from build123d import *

# Parameters (mm, degrees)
F0_R     = 1.5
F0_R_2   = 2.5
F1_DEPTH = 5
F2_R     = 2.5


with BuildPart() as f1:
    # F0 (on Front) → F1 (new body)
    with BuildSketch(Plane.XZ):
        with BuildLine():
            Line((-20, -25), (20, -25))
            ThreePointArc((20, -25), (27.071068, -22.071068), (30, -15))
            Line((30, -15), (30, 15))
            ThreePointArc((30, 15), (27.071068, 22.071068), (20, 25))
            Line((20, 25), (-20, 25))
            ThreePointArc((-20, 25), (-27.071068, 22.071068), (-30, 15))
            Line((-30, 15), (-30, -15))
            ThreePointArc((-30, -15), (-27.071068, -22.071068), (-20, -25))
        make_face()
        with Locations((-6, -20.123001)):
            Circle(F0_R, mode=Mode.SUBTRACT)
        with Locations((6, -20.123001)):
            Circle(F0_R, mode=Mode.SUBTRACT)
        with Locations((-10, 0)):
            Circle(F0_R_2, mode=Mode.SUBTRACT)
        with Locations((10, 0)):
            Circle(F0_R_2, mode=Mode.SUBTRACT)
    extrude(amount=F1_DEPTH)

    # F2
    f2_edges = [f1.edges().sort_by_distance(p)[0] for p in [
        (-30, -5, 0),
        (30, -5, 0),
        (0, -5, 25),
        (0, -5, -25),
        (-27.071068, -5, -22.071068),
        (27.071068, -5, -22.071068),
        (-27.071068, -5, 22.071068),
        (27.071068, -5, 22.071068),
    ]]
    fillet(f2_edges, radius=F2_R)


solid = f1.part
Work out the finished part from the listing and answer in its coordinate system (mm). Give positions to 0.01 mm unless a question says otherwise; leave off trailing zeros. Loops run counter-clockwise (first coordinate to the right, second up) from the corner with the lowest first, then second, coordinate; pieces in that order, holes last. Notation, with made-up numbers: (-32.75, 13.25) -> (7.25, 13.25) arc R19 cw to (7.25, 27.25) -> close; hole circle Ø1 at (7, -15). An arc over 180 degrees is marked (long way). Use a Markdown table: item, result. Add a question column.
1. Determine the mould class of faces 1 (the cylindrical face through (7.5, -2.5, 0.1)), 2 (the cylindrical face through (26.99, -1.23, -22.15)), 3 (the flat face through (0, -5, 0)) for opening direction X: released by +X, released by -X, zero draft, split by the parting line, or undercut.
2. Find the intervals of material crossed by probe 1 along Z at (x, y) = (-6, -2.6); probe 2 along X at (y, z) = (-1.8, -0.5); probe 3 along Z at (x, y) = (10, -1.75), in increasing order.
3. Section A-A on z = 0 is taken. Determine the outline of the cut face in (x, y).
4. Section D-D on y = -1.05 is taken. Determine the outline of the cut face in (x, z).
5. Section B-B on x = -6 is taken. Determine the outline of the cut face in (y, z).
6. A flat-ended cylindrical pin translates along its axis: pin 1 Ø1.5 at (y, z) = (-4.5, 5) entering from -X. Find the tip coordinate at first contact, or state that the pin passes through.
7. Section C-C on y = -4.05 is taken. Determine the outline of the cut face in (x, z).
Results below:
| question | item | result |
|---|---|---|
| 1 | face 1 | undercut |
| 1 | face 2 | released by +X |
| 1 | face 3 | zero draft |
| 2 | probe 1 | z = -25 to -21.62, -18.62 to 25 |
| 2 | probe 2 | x = -30 to -12.45, -7.55 to 7.55, 12.45 to 30 |
| 2 | probe 3 | z = -25 to -2.5, 2.5 to 25 |
| 3 | outline | (-30, -2.5) arc R2.5 ccw to (-27.5, -5) -> (-12.5, -5) -> (-12.5, 0) -> (-30, 0) -> close; (-7.5, -5) -> (7.5, -5) -> (7.5, 0) -> (-7.5, 0) -> close; (12.5, -5) -> (27.5, -5) arc R2.5 ccw to (30, -2.5) -> (30, 0) -> (12.5, 0) -> close |
| 4 | outline | (-30, -15) arc R10 ccw to (-20, -25) -> (20, -25) arc R10 ccw to (30, -15) -> (30, 15) arc R10 ccw to (20, 25) -> (-20, 25) arc R10 ccw to (-30, 15) -> close; hole circle Ø5 at (-10, 0); hole circle Ø3 at (-6, -20.12); hole circle Ø3 at (6, -20.12); hole circle Ø5 at (10, 0) |
| 5 | outline | (-5, -22.5) arc R2.5 ccw to (-2.5, -25) -> (0, -25) -> (0, -21.62) -> (-5, -21.62) -> close; (-5, -18.62) -> (0, -18.62) -> (0, 25) -> (-2.5, 25) arc R2.5 ccw to (-5, 22.5) -> close |
| 6 | pin 1 | stops at x = -29.67 |
| 7 | outline | (-29.46, -15) arc R9.46 ccw to (-20, -24.46) -> (20, -24.46) arc R9.46 ccw to (29.46, -15) -> (29.46, 15) arc R9.46 ccw to (20, 24.46) -> (-20, 24.46) arc R9.46 ccw to (-29.46, 15) -> close; hole circle Ø5 at (-10, 0); hole circle Ø3 at (-6, -20.12); hole circle Ø3 at (6, -20.12); hole circle Ø5 at (10, 0) |
